Autodesk Inventor part; units mm, degrees
ref_plane "YZ Plane" through (0, 0, 0) normal (1, 0, 0) x (0, 1, 0)
ref_plane "XZ Plane" through (0, 0, 0) normal (0, 1, 0) x (-1, 0, 0)
ref_plane "XY Plane" through (0, 0, 0) normal (0, 0, 1) x (1, 0, 0)
sketch "Эскиз1" plane through (0, 0, 0) normal (0, 1, 0) x (-1, 0, 0)
  arc A0 (46.7842, -80.4226) -> (85.3343, -22.1214) centre (-1.3087, -6.7268) ccw
  spline S0 degree 3 poles (85.3343, -22.1214) (85.7228, -19.9347) (86.0863, -17.3865) (86.5105, -12.698) (86.6278, -10.6493) (86.6714, -8.5984) (86.715, -6.5474) (86.685, -4.4956) (86.4606, 0.2067) (86.2058, 2.768) (85.9106, 4.9693) knots -3.249933 -3.249933 -3.249933 -3.249933 -2.410881 -2.410881 -1.809443 -1.809443 -1.809443 -1.208005 -1.208005 -0.368953 -0.368953 -0.368953 -0.368953
  arc A1 (85.9106, 4.9693) -> (-88.528, 4.9693) centre (-1.3087, -6.7268) ccw
  spline S1 degree 3 poles (-88.528, 4.9693) (-88.8231, 2.768) (-89.078, 0.2067) (-89.3023, -4.4956) (-89.3324, -6.5474) (-89.2888, -8.5984) (-89.2451, -10.6493) (-89.1279, -12.698) (-88.7037, -17.3865) (-88.3402, -19.9347) (-87.9517, -22.1214) knots -3.249933 -3.249933 -3.249933 -3.249933 -2.410881 -2.410881 -1.809443 -1.809443 -1.809443 -1.208005 -1.208005 -0.368953 -0.368953 -0.368953 -0.368953
  arc A2 (-87.9517, -22.1214) -> (-49.4016, -80.4226) centre (-1.3087, -6.7268) ccw
  line L0 (-48.3085, -80.7477) -> (45.6912, -80.7477)
  arc A3 (-49.4016, -80.4226) -> (-48.3085, -80.7477) centre (-48.3085, -78.7477) ccw
  arc A4 (45.6912, -80.7477) -> (46.7842, -80.4226) centre (45.6912, -78.7477) ccw
  circle A5 centre (53.4633, -41.7268) radius 20
  circle A6 centre (-56.0807, -41.7268) radius 20
  circle A7 centre (-36.3087, 48.0452) radius 20
  circle A8 centre (33.6913, 48.0452) radius 20
  circle A9 centre (-1.3087, -6.7268) radius 25
  circle A10 centre (70.6913, 17.2732) radius 3.25 construction
  circle A11 centre (-73.3087, 17.2732) radius 3.25 construction
  circle A12 centre (70.6913, 17.2732) radius 8
  circle A13 centre (-73.3087, 17.2732) radius 8
  point P0 (0, 0)
  dimension "d0" = 16
  dimension "d1" = 16
extrude "Выдавливание1" add sketch "Эскиз1" along normal blind 3
properties part number "vverh"
Source: CAD feature listing. Evaluate the final solid. Frame: model axes, mm. Give positions to 0.01 mm unless a question says otherwise; leave off trailing zeros. Write each loop counter-clockwise with the first axis right and the second up, starting at its lowest first coordinate (ties: lowest second). Pieces come first, ordered by that corner, then holes. Notation, with made-up numbers: (86, 20.25) -> (133, 20.25) arc R11 cw to (133, 39.25) -> close; hole circle Ø9 at (79.25, 33). An arc over 180 degrees is marked (long way). Return JSON: item names as keys, results as strings. Group by question number.
1. Section D-D, the plane y = 2.1. Count the separate pieces of the cut face and the enclosed holes in it, then the cut area to 3 significant figures.
2. Pin query (flat end, axial travel): pin 1 Ø24 at (x, z) = (-33.69, 48.05) entering from +Y; pin 2 Ø5 at (x, z) = (-51.5, 39.5) entering from -Y. Return the tip coordinate at first contact, or that it passes through.
3. Section A-A, the plane x = 69. Output: boundary loops of the cut face in (y, z).
4. Material intervals for line 1 (X direction, y = 1.75, z = 40.5); line 2 (Z direction, x = 21, y = 2.55); line 3 (X direction, y = 0.8, z = -49), sorted ascending. Write a range as from..to.
5. Mould query, pull axis X, two halves, no side actions, for faces 1 (the face through (-72.4, 1.5, -54.8)), 2 (the face through (3, 3, 19)), 3 (the face through (74.434, 1.479, -55.682)), 4 (the face through (-29.36, 1.48, 67.57)). Classes: +X half, -X half, draft (parallel to the pull), parting line (faces both ways), or undercut.
6. Section B-B, the plane z = 44. Output: boundary loops of the cut face in (x, y), then the cut area to 3 significant figures.
7. Section C-C, the plane x = -57.5. Output: boundary loops of the cut face in (y, z), then the cut area to 3 significant figures.
Determined:
{
 "1": {"separate pieces": "1", "enclosed holes": "7", "area": "16,000 mm2"},
 "2": {"pin 1": "passes through", "pin 2": "stops at y = 0"},
 "3": {"outline": "(0, -62.96) -> (3, -62.96) -> (3, -56.99) -> (0, -56.99) -> close; (0, -26.46) -> (3, -26.46) -> (3, 10.53) -> (0, 10.53) -> close; (0, 24.01) -> (3, 24.01) -> (3, 49.5) -> (0, 49.5) -> close"},
 "4": {"line 1": "x = -72.95..-52.21, -15.17..17.79, 54.83..75.56", "line 2": "z = -80.75..-22.13, 8.68..35.17, 60.92..79.04", "line 3": "x = -75.87..-72.09, -34.83..37.45, 74.71..78.49"},
 "5": {"face 1": "-X half", "face 2": "draft", "face 3": "+X half", "face 4": "undercut"},
 "6": {"outline": "(-70.6, 0) -> (-53.28, 0) -> (-53.28, 3) -> (-70.6, 3) -> close; (-14.1, 0) -> (16.72, 0) -> (16.72, 3) -> (-14.1, 3) -> close; (55.9, 0) -> (73.22, 0) -> (73.22, 3) -> (55.9, 3) -> close", "area": "196 mm2"},
 "7": {"outline": "(0, -72.19) -> (3, -72.19) -> (3, -61.32) -> (0, -61.32) -> close; (0, -22.14) -> (3, -22.14) -> (3, 58.74) -> (0, 58.74) -> close", "area": "275 mm2"}
}
